Geometry: final body of the model. Coordinates: model frame, mm. Face numbers are marked on the shaded views. A direction names the side the tool comes from. Coordinates: 2 decimals unless noted, no trailing zeros. Write each loop counter-clockwise with the first axis right and the second up, starting at its lowest first coordinate (ties: lowest second). Pieces come first, ordered by that corner, then holes. Notation, with made-up numbers: (84.25, -21) - (97.25, -21) arc R13 cw to (97.25, -7) - close; hole circle Ø8 at (83.5, 4.25). An arc over 180 degrees is marked (long way). Put each result on its own line as item: value.
```python
from build123d import *

# Parameters (mm, degrees)
F0_W     = 42.372167
F0_H     = 29.660501
F1_DEPTH = 152.4


with BuildPart() as f1:
    # F0 (on Front) → F1 (new body)
    with BuildSketch(Plane.XZ):
        with BuildLine():
            ThreePointArc((109.582473, 70.123763), (44.267725, 65.810023), (14.578056, 7.473514))
            Line((14.578056, 7.473514), (79.013996, 7.473514))
            ThreePointArc((79.013996, 7.473514), (87.094947, 30.642993), (109.582473, 40.463262))
            Line((109.582473, 40.463262), (109.582473, 70.123763))
        make_face()
        Polygon((14.578056, 7.473514), (-79.013996, 7.473514), (-79.013996, -7.473514), (79.013996, -7.473514), (79.013996, 7.473514), align=None)
        with Locations((130.768556, 55.293512)):
            Rectangle(F0_W, F0_H)
    extrude(amount=F1_DEPTH)


solid = f1.part
```
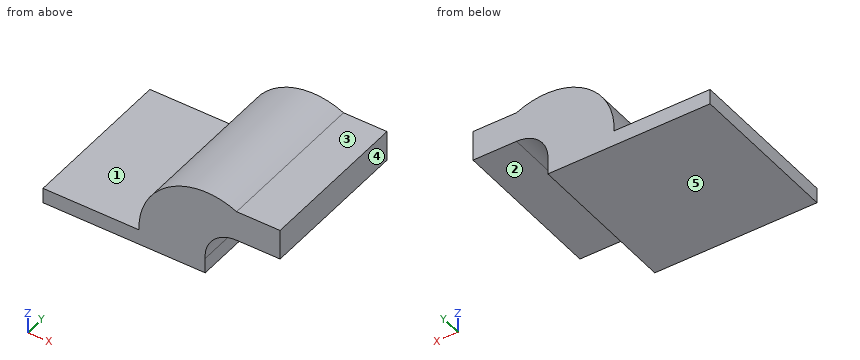
1. Pin query (flat end, axial travel): pin 1 Ø12.5 at (x, y) = (135, -56) entering from -Z; pin 2 Ø7.5 at (y, z) = (-86.5, 0.5) entering from +X; pin 3 Ø1 at (y, z) = (-128.5, 14.5) entering from -X. Return the tip coordinate at first contact, or that it passes through.
Answer below:
pin 1: stops at z = 40.46
pin 2: stops at x = 79.01
pin 3: stops at x = 14.6
2. Section query C-C (z = 66). Return loops of the section in (x, y).
Answer below:
outline: (44.56, -152.4) - (151.95, -152.4) - (151.95, 0) - (44.56, 0) - close
3. Ray query, probe 1 along Z at (x, y) = (135, -19); probe 2 along Z at (x, y) = (-17, -76); probe 3 along X at (y, z) = (-117.5, 1). Return the intervals inside material, ascending. Write a range as from..to.
Answer below:
probe 1: z = 40.46..70.12
probe 2: z = -7.47..7.47
probe 3: x = -79.01..79.01
4. Set-up query: the marked faces 1, 2, 3, 4 and 5. Return all of +Z, -Z, +X, -X, +Y, -Y with unobstructed straight access to the full face (end or side cutting, diameter ignored); none if empty.
Answer below:
face 1: +Z, -X, +Y, -Y
face 2: -Z, +X, +Y, -Y
face 3: +Z, +X, +Y, -Y
face 4: +Z, -Z, +X, +Y, -Y
face 5: -Z, +X, -X, +Y, -Y
5. Section query A-A (y = -107). Return loops of the section in (x, z).
Answer below:
outline: (-79.01, -7.47) - (79.01, -7.47) - (79.01, 7.47) arc R30.66 cw to (109.58, 40.46) - (151.95, 40.46) - (151.95, 70.12) - (109.58, 70.12) arc R66.21 ccw to (14.58, 7.47) - (-79.01, 7.47) - close
6. Section query B-B (x = 122). Return loops of the section in (y, z).
Answer below:
outline: (-152.4, 40.46) - (0, 40.46) - (0, 70.12) - (-152.4, 70.12) - close
